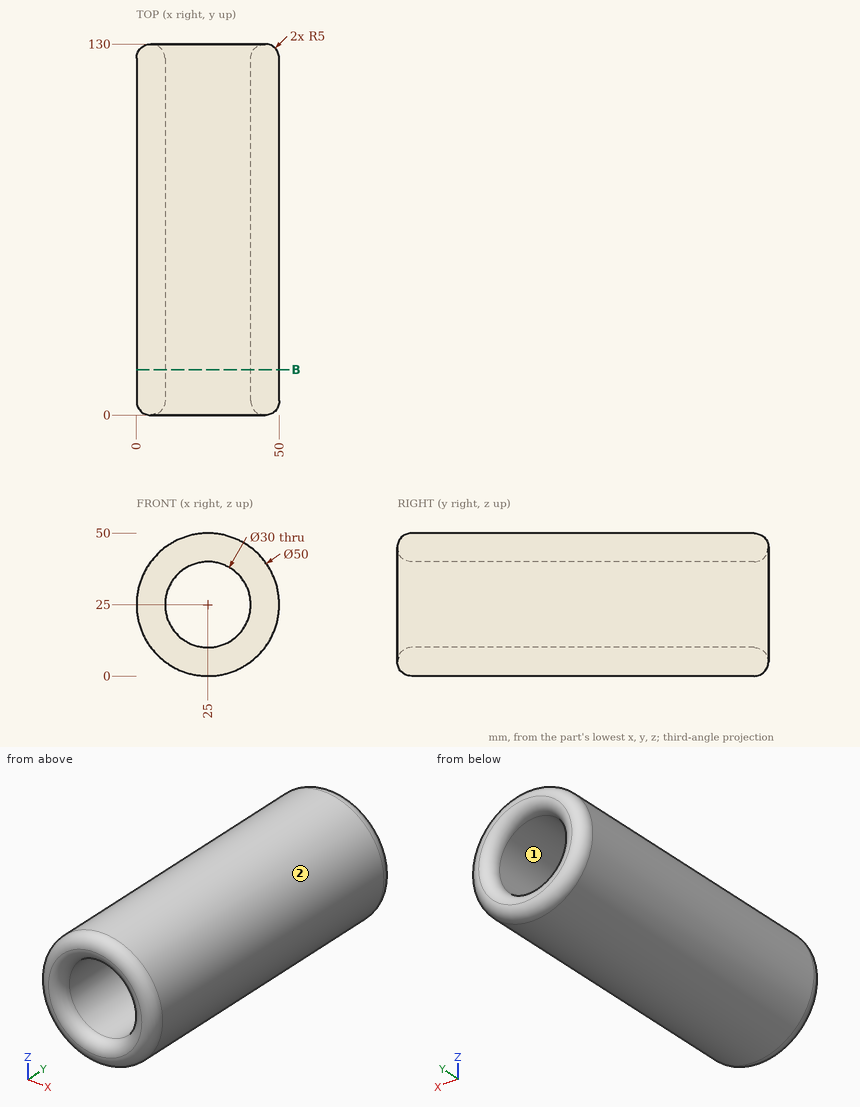
Here's the drawing with two shaded views (mm, measured from the low corner). I have some questions. Coordinates: 2 decimals unless noted, no trailing zeros. Order: outer loops, then holes, each group sorted by start corner. A loop starts at its lowest first (then second) coordinate and runs counter-clockwise, first axis right, second up.
Q1. Please list where these lines run through material, in increasing order: L1, parallel to Z at x = 25, y = 83; L2, parallel to Y at x = 5.5, z = 29; L3, parallel to X at y = 86.5, z = 28.
Q2. Thinking about a two-plate mould opening in Z: for the marked faces 1 and 2, which applies, released by +Z, released by -Z, zero draft, split by the parting line, or undercut?
Q3. Will these pins go through, and if not, where does the flat tip stop? pin 1 (1.5 mm diameter, centred on x = 18.5, y = 34, fed in from +Z); pin 2 (10 mm diameter, centred on x = 39, y = 46, fed in from +Z); pin 3 (1.5 mm diameter, centred on x = 5, y = 94, fed in from +Z).
Q4. Suppose I cut it at B-B on y = 16. Please give me the cut outline in (x, z).
Answer:
1. L1: z = 0 to 10, 40 to 50
1. L2: y = 0 to 130
1. L3: x = 0.18 to 10.3, 39.7 to 49.82
2. face 1: undercut
2. face 2: split by the parting line
3. pin 1: stops at z = 49.33
3. pin 2: stops at z = 48.32
3. pin 3: stops at z = 40.95
4. outline: circle Ø50 at (25, 25); hole circle Ø30 at (25, 25)
